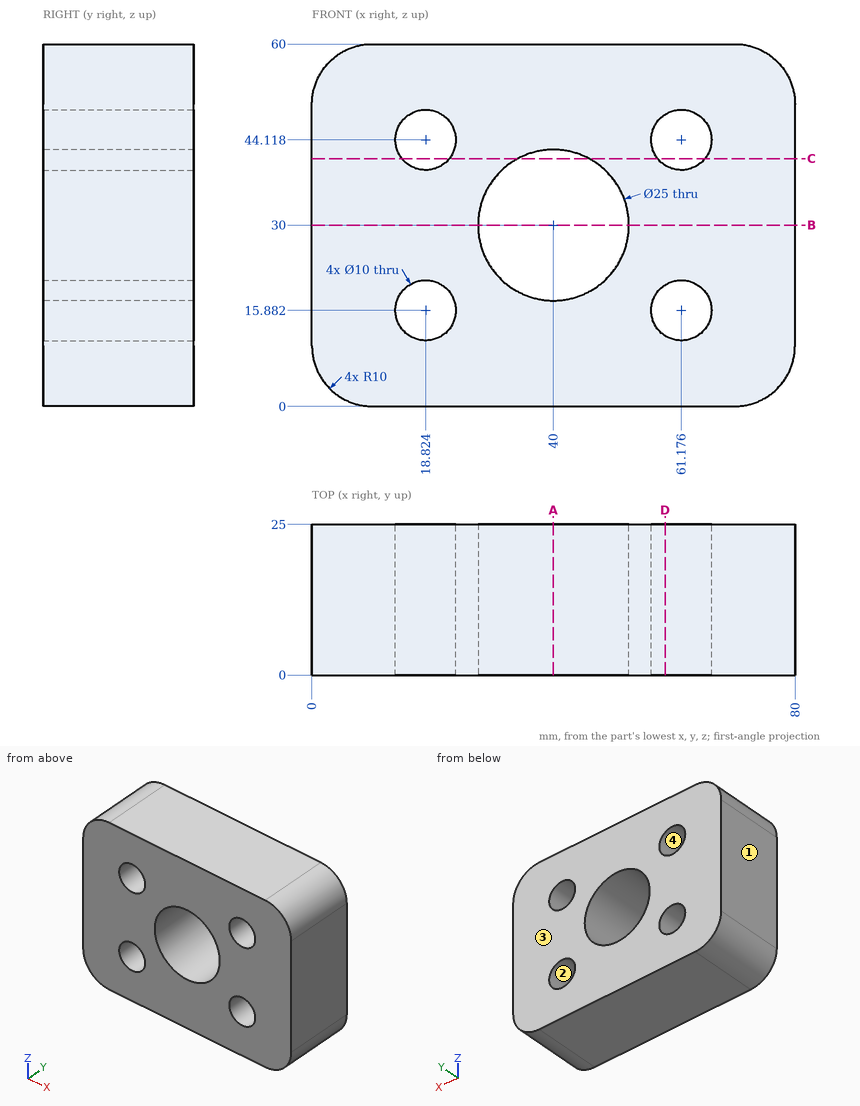
Can you work these out from the drawing? Everything is in mm from the part's minimum corner. Give positions to 0.01 mm unless a question says otherwise; leave off trailing zeros. Order: outer loops, then holes, each group sorted by start corner. A loop starts at its lowest first (then second) coordinate and runs counter-clockwise, first axis right, second up. Notation, with made-up numbers: M 53.25,69.5 L 75.25,69.5 A10 ccw 75.25,86.5 Z; hole C 82,21.25 d8. An arc over 180 degrees is marked long. Use a Markdown table: item, result. Add a question column.
1. For pin 1 Ø6 at (x, z) = (61.18, 44.12) entering from +Y, with a flat end and sliding along its axis, tell me the tip position at first contact or that it passes through.
2. Suppose I cut it at A-A (x = 40). List the corners of the cut face in (y, z) for me, and give its area (3 significant figures).
3. If we mould it in two halves opening along X, with no side actions, what happens to the marked faces 1, 2, 3 and 4? For each: +X half, -X half, draft (parallel to the pull), parting line (faces both ways), or undercut.
4. Suppose I cut it at C-C (z = 41). List the corners of the cut face in (x, y) for me (1 decimal), and give its area (3 significant figures).
5. Suppose I cut it at D-D (x = 58.5). List the corners of the cut face in (y, z) for me (1 decimal), and give its area (3 significant figures).
6. Suppose I cut it at B-B (z = 30). List the corners of the cut face in (x, y) for me, and give its area (4 significant figures).
7. I need wall thicknesses on probe 1 along X at (y, z) = (13.75, 43.5) (1 decimal); probe 2 along X at (y, z) = (11, 19) (1 decimal); probe 3 along X at (y, z) = (17.25, 44) (1 decimal). Which ranges of each line are inside material? Lowest first, please. Write a range as from..to.
Results list:
| question | item | result |
|---|---|---|
| 1 | pin 1 | passes through |
| 2 | outline | M 0,0 L 25,0 L 25,17.5 L 0,17.5 Z; M 0,42.5 L 25,42.5 L 25,60 L 0,60 Z |
| 2 | area | 875 mm² |
| 3 | face 1 | -X half |
| 3 | face 2 | undercut |
| 3 | face 3 | draft |
| 3 | face 4 | undercut |
| 4 | outline | M 0,0 L 14.9,0 L 14.9,25 L 0,25 Z; M 22.7,0 L 34.1,0 L 34.1,25 L 22.7,25 Z; M 45.9,0 L 57.3,0 L 57.3,25 L 45.9,25 Z; M 65.1,0 L 80,0 L 80,25 L 65.1,25 Z |
| 4 | area | 1,310 mm² |
| 5 | outline | M 0,0 L 25,0 L 25,11.7 L 0,11.7 Z; M 0,20.1 L 25,20.1 L 25,39.9 L 0,39.9 Z; M 0,48.3 L 25,48.3 L 25,60 L 0,60 Z |
| 5 | area | 1,080 mm² |
| 6 | outline | M 0,0 L 27.5,0 L 27.5,25 L 0,25 Z; M 52.5,0 L 80,0 L 80,25 L 52.5,25 Z |
| 6 | area | 1,375 mm² |
| 7 | probe 1 | x = 0..13.9, 23.8..56.2, 66.1..80 |
| 7 | probe 2 | x = 0..14.9, 22.7..34.1, 45.9..57.3, 65.1..80 |
| 7 | probe 3 | x = 0..13.8, 23.8..56.2, 66.2..80 |
